Read the model definition and answer for the solid it produces. Units are mm, in the model's axes. A direction names the side the tool comes from. Coordinates: 2 decimals unless noted, no trailing zeros. Write each loop counter-clockwise with the first axis right and the second up, starting at its lowest first coordinate (ties: lowest second). Pieces come first, ordered by that corner, then holes.
(1) Which of the six approach directions +Z, -Z, +X, -X, +Y, -Y give full straight-line access (tool end or side, diameter ignored) to faces 4 (the cylindrical face through (-0.69, 3.76, 3.1)), 5 (the cylindrical face through (-5.967, 4.573, 55.273)), 6 (the flat face through (-9, 4, 8.4)), 7 (the flat face through (8.21, 4, 38)), 8 (the flat face through (-2, 7.62, 30))?
(2) Given pin 1 (2.5 mm diameter, centred on y = 3.5, z = 14, fed in from -X); pin 2 (4 mm diameter, centred on y = 4.5, z = 46, fed in from +X); pin 3 (1.5 mm diameter, centred on x = -10.5, y = 3.5, fed in from -Z), each flat-ended and moving along its own axis, determine where each tip first touches the part or whether it passes through.
(3) The mould has two halves that part along Y. Classify faces 1 (the flat face through (-14.015, 4, 39)), 2 (the cylindrical face through (-5.967, 3.922, 12.213)), 3 (the flat face through (-2, 0, 30)): +Y half, -Y half, draft (parallel to the pull), parting line (faces both ways), or undercut.
(4) Find the intervals of material crossed by probe 1 along Z at (x, y) = (0, 3.75) (3 decimals); probe 2 along X at (y, z) = (2.25, 0) (3 decimals); probe 3 along Z at (x, y) = (1.75, 5), in increasing order.
(5) Section D-D on x = -8.25 is taken. Write down the section's boundary in (y, z).
(6) Section B-B on z = 0 is taken. Write down the section's boundary in (x, y) (3 decimals), then the cut area to 3 significant figures.
(7) Section A-A on x = 0 is taken. Write down the section's boundary in (y, z) (3 decimals).
(8) Section C-C on y = 4.5 is taken. Write down the section's boundary in (x, z) (3 decimals).
from build123d import *

# Parameters (mm, degrees)
SKETCH1_R           = 3.175
BOSS_EXTRUDE1_DEPTH = 7.62
SKETCH2_R           = 2.54
CUT_EXTRUDE1_DEPTH  = 6.35
SKETCH3_W           = 62.764867648
SKETCH3_H           = 7.62
SKETCH3_R           = 2.54
BOSS_EXTRUDE2_DEPTH = 9.525


with BuildPart() as part:
    # Sketch1 → Boss-Extrude1 (new body)
    with BuildSketch(Plane(origin=(0, 0, 0), x_dir=(1, 0, 0), z_dir=(0, 1, 0))):
        with BuildLine():
            Line((-4.490128061, -8.400260413), (-4.490128061, -71.165128061))
            Line((-4.490128061, -71.165128061), (8.209871939, -71.165128061))
            Line((8.209871939, -71.165128061), (8.209871939, -4.829454186))
            ThreePointArc((8.209871939, -4.829454186), (-2.578136518, 9.169451297), (-4.490128061, -8.400260413))
        make_face()
        Circle(SKETCH1_R, mode=Mode.SUBTRACT)
    extrude(amount=BOSS_EXTRUDE1_DEPTH)

    # Sketch2 → Cut-Extrude1 (cut)
    with BuildSketch(Plane.ZY.offset(4.490128061)):
        with Locations((14.750260413, 3.81)):
            Circle(SKETCH2_R)
        with Locations((52.850260413, 3.81)):
            Circle(SKETCH2_R)
    extrude(amount=-CUT_EXTRUDE1_DEPTH, mode=Mode.SUBTRACT)

    # Sketch3 → Boss-Extrude2 (add)
    with BuildSketch(Plane.ZY.offset(4.490128061)):
        with Locations((39.782694237, 3.81)):
            Rectangle(SKETCH3_W, SKETCH3_H)
        with Locations((52.850260413, 3.81)):
            Circle(SKETCH3_R, mode=Mode.SUBTRACT)
        with Locations((14.750260413, 3.81)):
            Circle(SKETCH3_R, mode=Mode.SUBTRACT)
    extrude(amount=BOSS_EXTRUDE2_DEPTH)


solid = part.part
Response:
1. face 4: +Y, -Y
1. face 5: -X
1. face 6: -X, +Y, -Y
1. face 7: +Z, +X, +Y, -Y
1. face 8: +Z, -Z, +X, -X, +Y
2. pin 1: stops at x = 1.86
2. pin 2: stops at x = 8.21
2. pin 3: stops at z = 8.4
3. face 1: draft
3. face 2: undercut
3. face 3: -Y half
4. probe 1: z = -9.525 to -3.175, 3.175 to 12.211, 17.29 to 50.311, 55.39 to 71.165
4. probe 2: x = -9.525 to -3.175, 3.175 to 9.525
4. probe 3: z = -9.36 to -2.65, 2.65 to 12.51, 16.99 to 50.61, 55.09 to 71.17
5. outline: (0, -4.76) - (7.62, -4.76) - (7.62, 4.76) - (0, 4.76) - close; (0, 8.4) - (7.62, 8.4) - (7.62, 71.17) - (0, 71.17) - close; hole circle Ø5.08 at (3.81, 14.75); hole circle Ø5.08 at (3.81, 52.85)
6. outline: (-9.525, 0) - (-3.175, 0) - (-3.175, 7.62) - (-9.525, 7.62) - close; (3.175, 0) - (9.525, 0) - (9.525, 7.62) - (3.175, 7.62) - close
6. area: 96.8 mm2
7. outline: (0, -9.525) - (7.62, -9.525) - (7.62, -3.175) - (0, -3.175) - close; (0, 3.175) - (7.62, 3.175) - (7.62, 71.165) - (0, 71.165) - close; hole circle Ø5.08 at (3.81, 14.75); hole circle Ø5.08 at (3.81, 52.85)
8. outline: (-14.015, 8.4) - (-4.49, 8.4) arc R9.525 ccw (long way) to (8.21, 4.829) - (8.21, 71.165) - (-14.015, 71.165) - (-14.015, 55.295) - (1.86, 55.295) - (1.86, 50.406) - (-14.015, 50.406) - (-14.015, 17.195) - (1.86, 17.195) - (1.86, 12.306) - (-14.015, 12.306) - close; hole circle Ø6.35 at (0, 0)
